```python
from build123d import *

# Parameters (mm, degrees)
SKIZZE3_R                             = 4.65
SCHNITT_LINEAR_AUSTRAGEN1_DEPTH       = 23
SKIZZE4_R                             = 2.5
SCHNITT_LINEAR_AUSTRAGEN2_DEPTH       = 32.476295332
AUFSATZ_LINEAR_AUSTRAGEN2_DEPTH       = 6
SKIZZE10_R                            = 2.1
SCHNITT_LINEAR_AUSTRAGEN4_DEPTH       = 6
SKIZZE13_W                            = 6
SKIZZE13_H                            = 0.905916259
AUFSATZ_LINEAR_AUSTRAGEN3_DEPTH       = 6
SKIZZE14_W                            = 6
SKIZZE14_H                            = 0.886770142
AUFSATZ_LINEAR_AUSTRAGEN4_DEPTH       = 6
AUFSATZ_LINEAR_AUSTRAGEN5_DEPTH       = 6
AUFSATZ_LINEAR_AUSTRAGEN6_DEPTH       = 6
SCHNITT_LINEAR_AUSTRAGEN5_DEPTH       = 1
KREISMUSTER1_COUNT                    = 4
AUFSATZ_LINEAR_AUSTRAGEN7_DEPTH       = 1
AUFSATZ_LINEAR_AUSTRAGEN7_DEPTH_BACK  = 7
SKIZZE24_R                            = 1.46260877
AUFSATZ_LINEAR_AUSTRAGEN8_DEPTH       = 1
AUFSATZ_LINEAR_AUSTRAGEN8_DEPTH_BACK  = 7
SKIZZE25_R                            = 0.941763398
AUFSATZ_LINEAR_AUSTRAGEN9_DEPTH       = 1
AUFSATZ_LINEAR_AUSTRAGEN9_DEPTH_BACK  = 7
SKIZZE26_R                            = 0.9041841
AUFSATZ_LINEAR_AUSTRAGEN10_DEPTH      = 1
AUFSATZ_LINEAR_AUSTRAGEN10_DEPTH_BACK = 7
SKIZZE27_R                            = 0.932524048
SKIZZE28_W                            = 1.499442475
SKIZZE28_H                            = 3.05198511
SCHNITT_LINEAR_AUSTRAGEN6_DEPTH       = 2
SKIZZE29_W                            = 1.472214026
SKIZZE29_H                            = 4.476539639
SCHNITT_LINEAR_AUSTRAGEN7_DEPTH       = 0.6


with BuildPart() as part:
    # Skizze2 → Rotation5 (revolve)
    with BuildSketch(Plane.XY, mode=Mode.PRIVATE) as rotation5_sk:
        Polygon((0, 0), (0, 6), (3.36648022, 10.528331662), (6.412062892, 8.264165831), (9.130397088, 11.920661045), (12.157026773, 9.06464462), (15.190566342, 12.27940236), (17.374944781, 9.800306185), (20.845408565, 12.858197338), (23.539774185, 9.800306185), (27.723555025, 13.486714461), (30.156102347, 10.725966298), (34.013267201, 14.124587063), (36.476289904, 11.329251761), (37.323543296, 15.194689333), (45.693256891, 15.194689333), (45.693256891, 0), (40, 0), align=None)
    revolve(rotation5_sk.sketch.rotate(Axis((45.693256891, 0, 0), (-1, 0, 0)), 90), axis=Axis((45.693256891, 0, 0), (-1, 0, 0)))

    # Skizze3 → Schnitt-Linear austragen1 (cut)
    with BuildSketch(Plane.ZY):
        Circle(SKIZZE3_R)
    extrude(amount=-SCHNITT_LINEAR_AUSTRAGEN1_DEPTH, mode=Mode.SUBTRACT)

    # Skizze4 → Schnitt-Linear austragen2 (cut, through all)
    with BuildSketch(Plane.ZY.offset(-23)):
        Circle(SKIZZE4_R)
    extrude(amount=-SCHNITT_LINEAR_AUSTRAGEN2_DEPTH, mode=Mode.SUBTRACT)

    # Skizze8 → Aufsatz-Linear austragen2 (add)
    with BuildSketch(Plane.ZY.offset(-20)):
        Polygon((5.135425827, 1.713216567), (16, 9.637964787), (16, 40), (14, 40), (14, 10.654654556), (3.956822965, 3.329043072), align=None)
    extrude(amount=-AUFSATZ_LINEAR_AUSTRAGEN2_DEPTH)

    # Skizze10 → Schnitt-Linear austragen4 (cut)
    with BuildSketch(Plane.XY.offset(16)):
        with Locations((23, 36)):
            Circle(SKIZZE10_R)
    extrude(amount=-SCHNITT_LINEAR_AUSTRAGEN4_DEPTH, mode=Mode.SUBTRACT)

    # Skizze13 → Aufsatz-Linear austragen3 (add)
    with BuildSketch(Plane(origin=(0, -1.326741748, 0.96774104), x_dir=(1, 0, 0), z_dir=(-4.115069899356744e-15, -0.8079132523298957, 0.5893014311112186))):
        with Locations((23, 13.484679747)):
            Rectangle(SKIZZE13_W, SKIZZE13_H)
    extrude(amount=AUFSATZ_LINEAR_AUSTRAGEN3_DEPTH)

    # Skizze14 → Aufsatz-Linear austragen4 (add)
    with BuildSketch(Plane(origin=(0, 0.289084756, -0.210861822), x_dir=(1, 0, 0), z_dir=(4.115069899356744e-15, 0.807913252329896, -0.5893014311112185))):
        with Locations((23, -13.507060971)):
            Rectangle(SKIZZE14_W, SKIZZE14_H)
    extrude(amount=AUFSATZ_LINEAR_AUSTRAGEN4_DEPTH)

    # Skizze16 → Aufsatz-Linear austragen5 (add)
    with BuildSketch(Plane(origin=(26, 0, 0), x_dir=(0, 0, -1), z_dir=(1, 0, 0))):
        Polygon((-15.763951974, 2.039248685), (-12.977538642, -11.010844393), (-12.386566519, -10.884661952), (-15.032050222, 1.505390937), align=None)
    extrude(amount=-AUFSATZ_LINEAR_AUSTRAGEN5_DEPTH)

    # Skizze17 → Aufsatz-Linear austragen6 (add)
    with BuildSketch(Plane(origin=(26, 0, 0), x_dir=(0, 0, -1), z_dir=(1, 0, 0))):
        Polygon((-6.807646475, 12.835007174), (4.174727727, 13.079302841), (4.174727727, 13.617814342), (-7.524079824, 13.357582087), align=None)
    extrude(amount=-AUFSATZ_LINEAR_AUSTRAGEN6_DEPTH)

    # Skizze19 → Schnitt-Linear austragen5 (cut)
    with BuildSketch(Plane(origin=(45.693256891, 0, 0), x_dir=(0, 0, -1), z_dir=(1, 0, 0))):
        Polygon((-1.799469686, 1.735485191), (-9.091569519, 0), (-1.799469686, -1.735485191), (-2.158394422, -1.261480685), (-2.415859445, -0.6431354), (-2.5, 0), (-2.408587239, 0.669856338), (-2.158394422, 1.261480685), align=None)
    schnitt_linear_austragen5 = extrude(amount=-SCHNITT_LINEAR_AUSTRAGEN5_DEPTH, mode=Mode.SUBTRACT)

    # Kreismuster1: Schnitt-Linear austragen5 ×4 about axis
    kreismuster1_axis = Axis((0, 0, 0), (1, 0, 0))
    for i in range(1, KREISMUSTER1_COUNT):
        add(schnitt_linear_austragen5.rotate(kreismuster1_axis, i * 360 / KREISMUSTER1_COUNT), mode=Mode.SUBTRACT)

    # Skizze24 → Aufsatz-Linear austragen7 (add, two sides: drawn at the far end of the back side and taken through both)
    with BuildSketch(Plane.ZY.offset(-20).offset(-AUFSATZ_LINEAR_AUSTRAGEN7_DEPTH_BACK)):
        with Locations(Location((11.453507252, 7.575434524, 0), (0, 0, 163.086563891))):
            Circle(SKIZZE24_R)
    extrude(amount=AUFSATZ_LINEAR_AUSTRAGEN7_DEPTH + AUFSATZ_LINEAR_AUSTRAGEN7_DEPTH_BACK)

    # Skizze25 → Aufsatz-Linear austragen8 (add, two sides: drawn at the far end of the back side and taken through both)
    with BuildSketch(Plane.ZY.offset(-20).offset(-AUFSATZ_LINEAR_AUSTRAGEN8_DEPTH_BACK)):
        with Locations((15.010107877, 10.189967275)):
            Circle(SKIZZE25_R)
    extrude(amount=AUFSATZ_LINEAR_AUSTRAGEN8_DEPTH + AUFSATZ_LINEAR_AUSTRAGEN8_DEPTH_BACK)

    # Skizze26 → Aufsatz-Linear austragen9 (add, two sides: drawn at the far end of the back side and taken through both)
    with BuildSketch(Plane(origin=(26, 0, 0), x_dir=(0, 0, -1), z_dir=(1, 0, 0)).offset(-AUFSATZ_LINEAR_AUSTRAGEN9_DEPTH_BACK)):
        with Locations((-7.144644053, 13.070033864)):
            Circle(SKIZZE26_R)
    extrude(amount=AUFSATZ_LINEAR_AUSTRAGEN9_DEPTH + AUFSATZ_LINEAR_AUSTRAGEN9_DEPTH_BACK)

    # Skizze27 → Aufsatz-Linear austragen10 (add, two sides: drawn at the far end of the back side and taken through both)
    with BuildSketch(Plane.ZY.offset(-20).offset(-AUFSATZ_LINEAR_AUSTRAGEN10_DEPTH_BACK)):
        with Locations((15.381369531, 1.80386132)):
            Circle(SKIZZE27_R)
    extrude(amount=AUFSATZ_LINEAR_AUSTRAGEN10_DEPTH + AUFSATZ_LINEAR_AUSTRAGEN10_DEPTH_BACK)

    # Skizze28 → Schnitt-Linear austragen6 (cut)
    with BuildSketch(Plane(origin=(0, -3.130195775, 14.660189045), x_dir=(1, 0, 0), z_dir=(-6.370898410720916e-15, -0.20881002467257814, 0.9779562227401783))):
        with Locations((22.790052948, -6.532291073)):
            Rectangle(SKIZZE28_W, SKIZZE28_H)
    extrude(amount=-SCHNITT_LINEAR_AUSTRAGEN6_DEPTH, mode=Mode.SUBTRACT)

    # Skizze29 → Schnitt-Linear austragen7 (cut)
    with BuildSketch(Plane(origin=(0, 13.518261299, 0.300704803), x_dir=(1, 0, 0), z_dir=(0, 0.9997526864415556, 0.022238838838681812))):
        with Locations((23.172580504, 2.23826982)):
            Rectangle(SKIZZE29_W, SKIZZE29_H)
    extrude(amount=-SCHNITT_LINEAR_AUSTRAGEN7_DEPTH, mode=Mode.SUBTRACT)


solid = part.part
```
Work out the finished part from the listing and answer in its coordinate system (mm). A direction names the side the tool comes from. Give positions to 0.01 mm unless a question says otherwise; leave off trailing zeros. Write each loop counter-clockwise with the first axis right and the second up, starting at its lowest first coordinate (ties: lowest second). Pieces come first, ordered by that corner, then holes. Notation, with made-up numbers: (51.25, 26.25) -> (69.25, 26.25) arc R32 cw to (69.25, 65.25) -> close; hole circle Ø2 at (9, 60.25). An arc over 180 degrees is marked (long way). Write item = value, one per line.
Q1. Section D-D on x = 32.5 is taken. Determine the outline of the cut face in (y, z).
Computed values:
outline = circle Ø25.58 at (0, 0); hole circle Ø5 at (0, 0)
Q2. A tool of negligible diameter and unlimited length cuts with its end or side. For faces 1 (the flat face through (27, 2, 15)), 2 (the flat face through (44.693, 0, -5)), 3 (the flat face through (22.958, 10.185, 8.741)), 4 (the conical face through (30.04, 10.6, 2.35)), 5 (the flat face through (22.96, 4.66, 13.85)), from which of +Z, -Z, +X, -X, +Y, -Y can it reach the whole face along a straight path? Write none if from no direction.
Computed values:
face_1 = +Z, +Y, -Y
face_2 = +X
face_3 = -X
face_4 = none
face_5 = +Z, -X
Q3. Section B-B on x = 39.5 is taken. Determine the outline of the cut face in (y, z), and give its area (3 significant figures).
Computed values:
outline = circle Ø30.39 at (0, 0); hole circle Ø5 at (0, 0)
area = 706 mm^2
Q4. Section A-A on y = 36 is taken. Determine the outline of the cut face in (x, z), and give its area (3 significant figures).
Computed values:
outline = (20, 14) -> (20.9, 14) -> (20.9, 16) -> (20, 16) -> close; (25.1, 14) -> (26, 14) -> (26, 16) -> (25.1, 16) -> close
area = 3.60 mm^2
Q5. For a pull along Y with two mould halves and no side action, classify faces 6 (the flat face through (22.958, 9.843, 12.888)), 7 (the cylindrical face through (11.34, 3.92, 2.5)), 8 (the cylindrical face through (41.57, -10.27, 11.2)) as pulls with the +Y half, pulls with the -Y half, needs draft (parallel to the pull), parting line crosses it, or undercut.
Computed values:
face_6 = pulls with the +Y half
face_7 = undercut
face_8 = parting line crosses it
Q6. Flat-ended cylindrical pins translate along their axes: pin 1 Ø1.3 at (y, z) = (6.5, 10) entering from -X; pin 2 Ø0.6 at (y, z) = (2, 15) entering from -X; pin 3 Ø1 at (x, y) = (38.5, -8.5) entering from -Z. Find the tip coordinate at first contact, or state that the pin passes through.
Computed values:
pin_1 = 8.65
pin_2 = 19
pin_3 = -12.92
Q7. Section C-C on y = 23 is taken. Determine the outline of the cut face in (x, z).
Computed values:
outline = (20, 14) -> (26, 14) -> (26, 16) -> (20, 16) -> close
Q8. Consider line 1 along X through (y, z) = (-12.5, -1); line 2 along X through (y, z) = (27, 15); line 3 along X through (y, z) = (10.5, 3) (1 decimal). Determine where each line is inside the solid, lowest interval first.
Computed values:
line_1 = 20.48 to 21.13, 26.65 to 28.56, 32.21 to 35.41, 36.74 to 45.69
line_2 = 20 to 26
line_3 = 8.4 to 10.2, 13.9 to 16.4, 18.6 to 22.6, 24.8 to 30, 30.4 to 45.7
